Can you work these out from the model? Positions are in its coordinate system, mm. A direction names the side the tool comes from. Coordinates: 2 decimals unless noted, no trailing zeros. Order: outer loops, then holes, each group sorted by start corner. A loop starts at its lowest first (then second) coordinate and runs counter-clockwise, first axis right, second up. Notation, with made-up numbers: (46, 80.5) -> (85, 80.5) arc R15 ccw to (85, 91.5) -> close; hole circle Ø2 at (82.5, 14.25). An arc over 180 degrees is marked (long way). Return JSON: item names as keys, results as strings. Group by question number.
1) If we section it at A-A, the plane y = -7.63: Please give me the cut outline in (x, z).
2) If we section it at D-D, the plane y = -11: Please give me the cut outline in (x, z), then the cut area to 3 significant figures.
3) If we section it at B-B, the plane x = -20.33: Please give me the cut outline in (y, z), then the cut area to 3 significant figures.
4) For faces 4 (the cylindrical face through (-18.346, -14.573, 4.929)), 5 (the flat face through (-6, -3.5, -2)), 6 (the flat face through (-13, 0, 5)), which set-ups out of +Z, -Z, +X, -X, +Y, -Y let a thin tool reach every point of the face, with its end or its side?
5) If we section it at C-C, the plane z = 9.5: Please give me the cut outline in (x, y).
6) If I drill on probe 1 along Z at (x, y) = (-9.5, -1.5); probe 2 along X at (y, z) = (4.5, 6.55); probe 3 along X at (y, z) = (-8, -2.25), over which ranges is the centre line in solid material (lowest first)? Write a range as from..to.
7) Thinking about a two-plate mould opening in Z: for faces 1 (the cylindrical face through (2.96, -7.09, 4.01)), 2 (the flat face through (-12.7, -13, 3)), 3 (the flat face through (-11, -5, 16.9)), which applies, +Z half, -Z half, draft (parallel to the pull), parting line (faces both ways), or undercut?
8) For pin 1 (12 mm diameter, centred on x = -5, z = 11, fed in from -Y); pin 2 (4.5 mm diameter, centred on x = -9, z = -2.5, fed in from -Y); pin 3 (1.2 mm diameter, centred on y = -4, z = -1.5, fed in from -X), each with a flat end and sliding along its axis, tell me the tip position at first contact or that it passes through.
from build123d import *

# Parameters (mm, degrees)
BOSS_EXTRUDE1_DEPTH = 12.9
SKETCH2_R           = 2.5
CUT_EXTRUDE1_DEPTH  = 38.288201887
SKETCH3_R           = 2.5
CUT_EXTRUDE2_DEPTH  = 38.288201887
SKETCH5_W           = 36
SKETCH5_H           = 24
BOSS_EXTRUDE3_DEPTH = 4
SKETCH6_W           = 17.3
SKETCH6_H           = 5.3
BOSS_EXTRUDE4_DEPTH = 12.9
SKETCH7_R           = 2.5
CUT_EXTRUDE3_DEPTH  = 40.182904435
EXTRUDE_3_DEPTH     = 4
SKETCH_5_W          = 3
SKETCH_5_H          = 20.9
CUT_EXTRUDE_1_DEPTH = 42.971537975
CUT_EXTRUDE_2_DEPTH = 4
SKETCH_7_W          = 16.9
SKETCH_7_H          = 1.5
CUT_EXTRUDE_3_DEPTH = 20
CUT_EXTRUDE5_REACH  = 40.998
SKETCH8_W           = 1.3
SKETCH8_H           = 12.9
SKETCH_9_W          = 4
SKETCH_9_H          = 24
CUT_EXTRUDE_4_DEPTH = 42.214196583
SKETCH_11_W         = 16.9
SKETCH_11_H         = 1.5
CUT_EXTRUDE_6_DEPTH = 32.774360733
SKETCH_13_W         = 12.9
SKETCH_13_H         = 3.8
EXTRUDE_5_DEPTH     = 1.3
EXTRUDE_6_DEPTH     = 4


with BuildPart() as part:
    # Sketch1 → Boss-Extrude1 (new body)
    with BuildSketch(Plane.XY):
        Polygon((-30, 0), (-30, 6), (6, 6), (6, -18), (0, -18), (0, 0), align=None)
    extrude(amount=BOSS_EXTRUDE1_DEPTH)

    # Sketch2 → Cut-Extrude1 (cut, through all)
    with BuildSketch(Plane.XZ):
        with Locations(Location((-20.33, 6.55, 0), (0, 0, 270))):
            Circle(SKETCH2_R)
    extrude(amount=-CUT_EXTRUDE1_DEPTH, mode=Mode.SUBTRACT)

    # Sketch3 → Cut-Extrude2 (cut, through all)
    with BuildSketch(Plane.ZY):
        with Locations(Location((6.45, -7.63, 0), (0, 0, 270))):
            Circle(SKETCH3_R)
    extrude(amount=-CUT_EXTRUDE2_DEPTH, mode=Mode.SUBTRACT)

    # Sketch5 → Boss-Extrude3 (add)
    with BuildSketch(Plane.XY.offset(12.9)):
        with Locations((-12, -6)):
            Rectangle(SKETCH5_W, SKETCH5_H)
    extrude(amount=BOSS_EXTRUDE3_DEPTH)

    # Sketch6 → Boss-Extrude4 (add)
    with BuildSketch(Plane(origin=(0, 0, 12.9), x_dir=(-1, 0, 0), z_dir=(0, 0, -1))):
        with Locations((21.35, -15.35)):
            Rectangle(SKETCH6_W, SKETCH6_H)
    extrude(amount=BOSS_EXTRUDE4_DEPTH)

    # Sketch7 → Cut-Extrude3 (cut, through all)
    with BuildSketch(Plane(origin=(0, -12.7, 0), x_dir=(1, 0, 0), z_dir=(0, 1, 0))):
        with Locations(Location((-20.33, -6.45, 0), (0, 0, 180))):
            Circle(SKETCH7_R)
    extrude(amount=-CUT_EXTRUDE3_DEPTH, mode=Mode.SUBTRACT)

    # 草图4 → 凸台-拉伸3 (add)
    with BuildSketch(Plane(origin=(0, 0, 0), x_dir=(-1, 0, 0), z_dir=(0, 0, -1))):
        Polygon((30, 6), (9, 6), (9, -4), (11, -4), (11, -18), (30, -18), align=None)
    extrude(amount=EXTRUDE_3_DEPTH)

    # 草图5 → 切除-拉伸1 (cut, through all)
    with BuildSketch(Plane.XZ.offset(18)):
        with Locations((-28.5, 6.45)):
            Rectangle(SKETCH_5_W, SKETCH_5_H)
    extrude(amount=-CUT_EXTRUDE_1_DEPTH, mode=Mode.SUBTRACT)

    # 草图6 → 切除-拉伸2 (cut)
    with BuildSketch(Plane(origin=(0, 0, -4), x_dir=(-1, 0, 0), z_dir=(0, 0, -1))):
        Polygon((11, -18), (11, -14), (13.1, -18), align=None)
    extrude(amount=-CUT_EXTRUDE_2_DEPTH, mode=Mode.SUBTRACT)

    # 草图7 → 切除-拉伸3 (cut)
    with BuildSketch(Plane(origin=(6, 0, 0), x_dir=(0, 0, -1), z_dir=(1, 0, 0))):
        with Locations((-8.45, -17.25)):
            Rectangle(SKETCH_7_W, SKETCH_7_H)
    extrude(amount=-CUT_EXTRUDE_3_DEPTH, mode=Mode.SUBTRACT)

    # Sketch8 → Cut-Extrude5 (cut, up to next)
    with BuildSketch(Plane.XZ.offset(16.5), mode=Mode.PRIVATE) as cut_extrude5_sk1:
        with Locations((-13.35, 6.45)):
            Rectangle(SKETCH8_W, SKETCH8_H)
    cut_extrude5_tool1 = extrude(cut_extrude5_sk1.sketch, amount=-CUT_EXTRUDE5_REACH, mode=Mode.PRIVATE) & part.part
    add(cut_extrude5_tool1.solids().sort_by_distance((-13.35, -16.5, 6.45))[0], mode=Mode.SUBTRACT)

    # 草图9 → 切除-拉伸4 (cut, through all)
    with BuildSketch(Plane(origin=(6, 0, 0), x_dir=(0, 0, -1), z_dir=(1, 0, 0))):
        with Locations((2, -6)):
            Rectangle(SKETCH_9_W, SKETCH_9_H)
    extrude(amount=-CUT_EXTRUDE_4_DEPTH, mode=Mode.SUBTRACT)

    # 草图11 → 切除-拉伸6 (cut, through all)
    with BuildSketch(Plane(origin=(-14, 0, 0), x_dir=(0, 0, -1), z_dir=(1, 0, 0))):
        with Locations((-8.45, -17.25)):
            Rectangle(SKETCH_11_W, SKETCH_11_H)
    extrude(amount=-CUT_EXTRUDE_6_DEPTH, mode=Mode.SUBTRACT)

    # 草图13 → 凸台-拉伸5 (add)
    with BuildSketch(Plane(origin=(-14, 0, 0), x_dir=(0, 0, -1), z_dir=(1, 0, 0))):
        with Locations((-6.45, -14.6)):
            Rectangle(SKETCH_13_W, SKETCH_13_H)
    extrude(amount=EXTRUDE_5_DEPTH)

    # 草图17 → 凸台-拉伸6 (add)
    with BuildSketch(Plane(origin=(0, 0, 0), x_dir=(-1, 0, 0), z_dir=(0, 0, -1))):
        Polygon((27, 6), (-6, 6), (-6, -16.5), (0, -16.5), (0, -3.5), (12.7, -3.5), (12.7, -16.5), (27, -16.5), (27, -12.7), (16.2, -12.7), (16.2, 0), (27, 0), align=None)
    extrude(amount=EXTRUDE_6_DEPTH)


solid = part.part
Result sheet:
{
 "1": {"outline": "(-27, 12.9) -> (0, 12.9) -> (0, 8.95) -> (6, 8.95) -> (6, 16.9) -> (-27, 16.9) -> close; (-16.2, -4) -> (-12.7, -4) -> (-12.7, 0) -> (-16.2, 0) -> close; (0, -4) -> (6, -4) -> (6, 3.95) -> (0, 3.95) -> close"},
 "2": {"outline": "(-27, 12.9) -> (0, 12.9) -> (0, -4) -> (6, -4) -> (6, 16.9) -> (-27, 16.9) -> close; (-16.2, -4) -> (-12.7, -4) -> (-12.7, 0) -> (-16.2, 0) -> close", "area": "247 mm2"},
 "3": {"outline": "(-16.5, -4) -> (-12.7, -4) -> (-12.7, 3.95) -> (-16.5, 3.95) -> close; (-16.5, 8.95) -> (-12.7, 8.95) -> (-12.7, 12.9) -> (0, 12.9) -> (0, 9.05) -> (6, 9.05) -> (6, 16.9) -> (-16.5, 16.9) -> close; (0, -4) -> (6, -4) -> (6, 4.05) -> (0, 4.05) -> close", "area": "207 mm2"},
 "4": {"face 4": "-Y", "face 5": "-Z, -Y", "face 6": "-X"},
 "5": {"outline": "(-27, -16.5) -> (-12.7, -16.5) -> (-12.7, -12.7) -> (-27, -12.7) -> close; (-27, 0) -> (0, 0) -> (0, -16.5) -> (6, -16.5) -> (6, 6) -> (-27, 6) -> close"},
 "6": {"probe 1": "z = -4..0, 12.9..16.9", "probe 2": "x = -27..-22.83, -17.83..6", "probe 3": "x = -16.2..-12.7, 0..6"},
 "7": {"face 1": "undercut", "face 2": "draft", "face 3": "+Z half"},
 "8": {"pin 1": "stops at y = -16.5", "pin 2": "stops at y = -3.5", "pin 3": "stops at x = -16.2"}
}
